```python
from build123d import *

# Parameters (mm, degrees)
SKETCH_1_R      = 7.5
SKETCH_1_R_2    = 3
SKETCH_1_W      = 32
SKETCH_1_H      = 15
SKETCH_1_R_3    = 1.6
EXTRUDE_1_DEPTH = 3
FILLET_1_R      = 3


with BuildPart() as part:
    # 草图1 → 凸台-拉伸1 (new body)
    # profile 1 of 3: a face of its own
    with BuildSketch(Plane(origin=(0, 0, 0), x_dir=(1, 0, 0), z_dir=(0, 1, 0))):
        with Locations((-22.85, -3.86)):
            Circle(SKETCH_1_R)
        with Locations(Location((-22.85, -3.86, 0), (0, 0, 270))):
            Circle(SKETCH_1_R_2, mode=Mode.SUBTRACT)
    # profile 2 of 3: a face of its own
    with BuildSketch(Plane(origin=(0, 0, 0), x_dir=(1, 0, 0), z_dir=(0, 1, 0))):
        with BuildLine():
            Line((0, 0), (0, 15))
            Line((0, 15), (-26.004488854, 2.944351554))
            ThreePointArc((-26.004488854, 2.944351554), (-18.813210831, 2.460944012), (-15.35, -3.86))
            ThreePointArc((-15.35, -3.86), (-17.02696903, -8.586765312), (-21.307949418, -11.199760214))
            Line((-21.307949418, -11.199760214), (32, 0))
            Line((32, 0), (0, 0))
        make_face()
    # profile 3 of 3: a face of its own
    with BuildSketch(Plane(origin=(0, 0, 0), x_dir=(1, 0, 0), z_dir=(0, 1, 0))):
        with Locations((16, 7.5)):
            Rectangle(SKETCH_1_W, SKETCH_1_H)
        with Locations(Location((26, 7.5, 0), (0, 0, 270))):
            Circle(SKETCH_1_R_3, mode=Mode.SUBTRACT)
        with Locations(Location((6, 7.5, 0), (0, 0, 270))):
            Circle(SKETCH_1_R_3, mode=Mode.SUBTRACT)
    extrude(amount=EXTRUDE_1_DEPTH)

    # 圆角1
    fillet_1_edges = [part.edges().sort_by_distance(p)[0] for p in [
        (0, 1.5, -15),
        (32, 1.5, -15),
        (32, 1.5, 0),
    ]]
    fillet(fillet_1_edges, radius=FILLET_1_R)


solid = part.part
```
Part model, mm, in its own coordinate system. Round coordinates to 2 decimals unless told otherwise and drop trailing zeros. Loops run counter-clockwise (first coordinate to the right, second up) from the corner with the lowest first, then second, coordinate; pieces in that order, holes last. Notation, with made-up numbers: (54, -33.5) -> (78, -33.5) arc R28 cw to (78, -5.5) -> close; hole circle Ø9 at (-16, 23.25). An arc over 180 degrees is marked (long way). Use a Markdown table: item, result.
1) Cut at B-B, the plane x = -22.85. List the corners of the cut face in (y, z), and give its area (3 significant figures).
The answers:
| item | result |
|---|---|
| outline | (0, -4.41) -> (3, -4.41) -> (3, 0.86) -> (0, 0.86) -> close; (0, 6.86) -> (3, 6.86) -> (3, 11.36) -> (0, 11.36) -> close |
| area | 29.3 mm2 |
2) Cut at D-D, the plane z = -7.5. List the corners of the cut face in (x, y), and give its area (3 significant figures).
The answers:
| item | result |
|---|---|
| outline | (-16.18, 0) -> (4.4, 0) -> (4.4, 3) -> (-16.18, 3) -> close; (7.6, 0) -> (24.4, 0) -> (24.4, 3) -> (7.6, 3) -> close; (27.6, 0) -> (32, 0) -> (32, 3) -> (27.6, 3) -> close |
| area | 125 mm2 |
3) Pull direction Z, two halves, no side cores. Call faces 1 (the flat face through (3.798, 1.479, 5.925)), 2 (the cylindrical face through (4.44, 1.48, -7.85)), 3 (the cylindrical face through (31.1, 1.52, -14.14)): pulls with the +Z half, pulls with the -Z half, needs draft (parallel to the pull), parting line crosses it, or undercut.
The answers:
| item | result |
|---|---|
| face 1 | pulls with the +Z half |
| face 2 | undercut |
| face 3 | pulls with the -Z half |
4) Drop a flat-ended pin along its axis: pin 1 Ø1.5 at (y, z) = (2.5, 2.5) entering from -X. Give the stop position or say it passes through.
The answers:
| item | result |
|---|---|
| pin 1 | stops at x = -30.33 |
5) Cut at C-C, the plane y = 2.15. List the corners of the cut face in (x, z).
The answers:
| item | result |
|---|---|
| outline | (-26, -2.94) -> (-0.6, -14.72) arc R3 ccw to (0.66, -15) -> (29, -15) arc R3 ccw to (32, -12) -> (32, -2.44) arc R3 ccw to (29.62, 0.5) -> (-21.31, 11.2) arc R7.5 ccw to start; hole circle Ø6 at (-22.85, 3.86); hole circle Ø3.2 at (6, -7.5); hole circle Ø3.2 at (26, -7.5) |
6) Cut at A-A, the plane z = 2. List the corners of the cut face in (x, y).
The answers:
| item | result |
|---|---|
| outline | (-30.12, 0) -> (-25.2, 0) -> (-25.2, 3) -> (-30.12, 3) -> close; (-20.5, 0) -> (22.48, 0) -> (22.48, 3) -> (-20.5, 3) -> close |
7) Probe line 1 (X direction, y = 2.3, z = -7.5); line 2 (X direction, y = 1.95, z = -8.75); line 3 (X direction, y = 0.85, z = -3). List the from-to ranges inside material, lowest first. Write a range as [from, to].
The answers:
| item | result |
|---|---|
| line 1 | x = [-16.18, 4.4], [7.6, 24.4], [27.6, 32] |
| line 2 | x = [-13.48, 5], [7, 25], [27, 32] |
| line 3 | x = [-25.88, 32] |
